Answer from the drawing. Dimensions are ordinates in mm from the lowest x, y and z of the part. A direction names the side the tool comes from. Coordinates: 2 decimals unless noted, no trailing zeros. Loops run counter-clockwise (first coordinate to the right, second up) from the corner with the lowest first, then second, coordinate; pieces in that order, holes last.
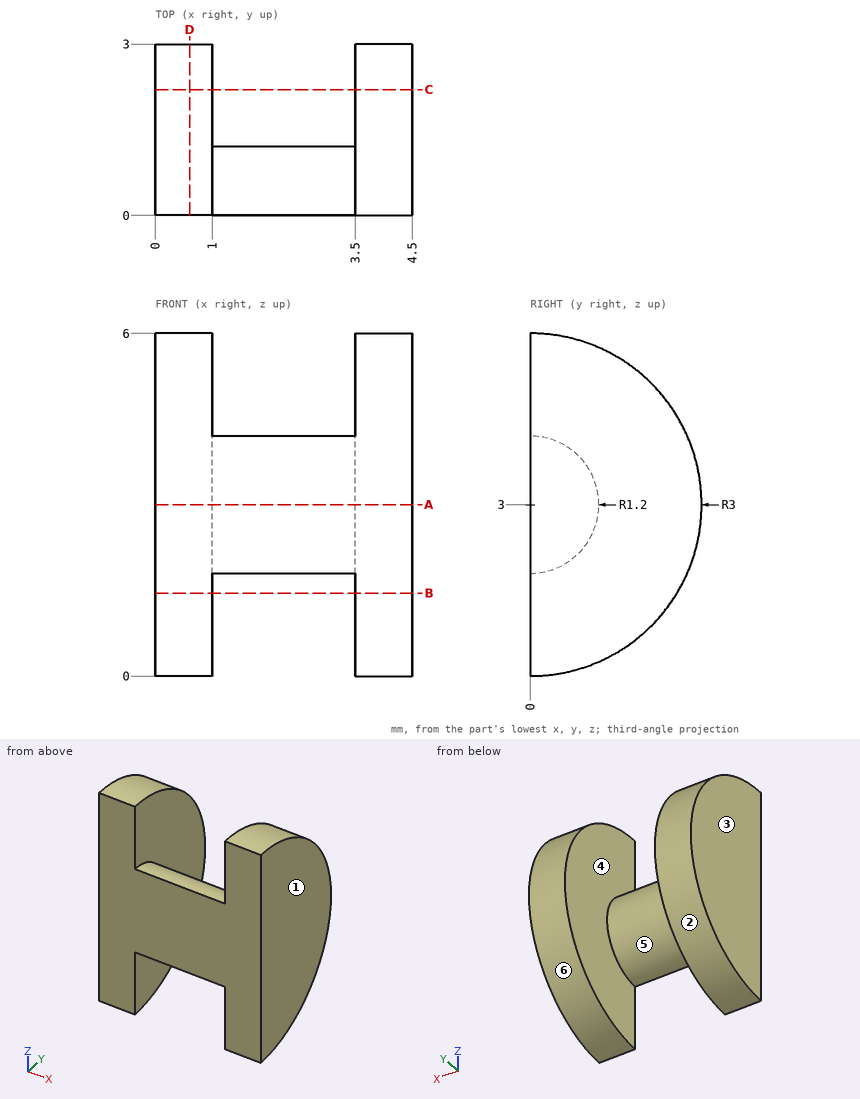
Item 1: A cutting plane is placed at A-A on z = 3. Determine the outline of the cut face in (x, y).
Numbers:
outline: (0, 0) - (4.5, 0) - (4.5, 3) - (3.5, 3) - (3.5, 1.2) - (1, 1.2) - (1, 3) - (0, 3) - close
Item 2: Find the intervals of material crossed by line 1 along X through (y, z) = (0.5, 4.75); line 2 along Y through (x, z) = (4.05, 0.6); line 3 along Y through (x, z) = (0.75, 1), in increasing order.
Numbers:
line 1: x = 0 to 1, 3.5 to 4.5
line 2: y = 0 to 1.8
line 3: y = 0 to 2.24
Item 3: A cutting plane is placed at C-C on y = 2.2. Determine the outline of the cut face in (x, z), then the cut area to 3 significant figures.
Numbers:
outline: (0, 0.96) - (1, 0.96) - (1, 5.04) - (0, 5.04) - close; (3.5, 0.96) - (4.5, 0.96) - (4.5, 5.04) - (3.5, 5.04) - close
area: 8.16 mm2
Item 4: A cutting plane is placed at B-B on z = 1.45. Determine the outline of the cut face in (x, y).
Numbers:
outline: (0, 0) - (1, 0) - (1, 2.57) - (0, 2.57) - close; (3.5, 0) - (4.5, 0) - (4.5, 2.57) - (3.5, 2.57) - close
Item 5: A cutting plane is placed at D-D on x = 0.6. Determine the outline of the cut face in (y, z).
Numbers:
outline: (0, 0) arc R3 ccw to (0, 6) - close
Item 6: Determine the mould class of the marked faces 1, 2, 3 and 4 for opening direction X: released by +X, released by -X, zero draft, split by the parting line, or undercut.
Numbers:
face 1: released by +X
face 2: zero draft
face 3: released by -X
face 4: undercut
Item 7: Which of the six approach directions +Z, -Z, +X, -X, +Y, -Y give full straight-line access (tool end or side, diameter ignored) to the marked faces 5 and 6?
Numbers:
face 5: +Y
face 6: +X, -X, +Y
